```python
from build123d import *

# Parameters (mm, degrees)
SKETCH1_W       = 1193.8
SKETCH1_H       = 1371.6
EXTRUDE1_DEPTH  = 635
EXTRUDE4_DEPTH  = 1270
SKETCH6_W       = 25.4
SKETCH6_H       = 25.4
EXTRUDE5_DEPTH  = 584.2
SKETCH8_W       = 25.4
SKETCH8_H       = 25.4
EXTRUDE6_DEPTH  = 1143
SKETCH9_W       = 25.4
SKETCH9_H       = 25.4
EXTRUDE7_DEPTH  = 584.2
SKETCH10_W      = 25.4
SKETCH10_H      = 25.4
EXTRUDE8_DEPTH  = 1143
SHELL2_T        = -25.4
SKETCH17_R      = 3.175
EXTRUDE14_DEPTH = 1927.050362789
SKETCH24_W      = 1143
SKETCH24_H      = 584.2
EXTRUDE15_DEPTH = 25.4
SKETCH12_W      = 1143
SKETCH12_H      = 76.2
EXTRUDE16_DEPTH = 38.1
SKETCH13_W      = 584.2
SKETCH13_H      = 76.2
EXTRUDE17_DEPTH = 38.1
SKETCH14_W      = 1143
SKETCH14_H      = 76.2
EXTRUDE18_DEPTH = 38.1
SKETCH11_W      = 584.2
SKETCH11_H      = 76.2
EXTRUDE19_DEPTH = 38.1
SKETCH30_W      = 1143
SKETCH30_H      = 5.614753794
EXTRUDE20_DEPTH = 76.2


with BuildPart() as part:
    # Sketch1 → Extrude1 (new body)
    with BuildSketch(Plane.XY):
        with Locations((596.9, 685.8)):
            Rectangle(SKETCH1_W, SKETCH1_H)
    extrude(amount=EXTRUDE1_DEPTH)

    # Sketch2 → Extrude4 (cut)
    with BuildSketch(Plane(origin=(0, 1371.6, 0), x_dir=(1, 0, 0), z_dir=(0, 1, 0))):
        Polygon((25.4, -609.6), (25.4, -635), (1168.4, -635), (1168.4, -609.6), (1193.8, -609.6), (1193.8, -25.4), (1168.4, -25.4), (1168.4, 0), (25.4, 0), (25.4, -25.4), (0, -25.4), (0, -609.6), align=None)
    extrude(amount=-EXTRUDE4_DEPTH, mode=Mode.SUBTRACT)

    # Sketch6 → Extrude5 (add)
    with BuildSketch(Plane.XY.offset(25.4)):
        with Locations((12.7, 1358.9)):
            Rectangle(SKETCH6_W, SKETCH6_H)
    extrude(amount=EXTRUDE5_DEPTH)

    # Sketch8 → Extrude6 (add)
    with BuildSketch(Plane(origin=(25.4, 0, 0), x_dir=(0, 0, -1), z_dir=(1, 0, 0))):
        with Locations((-622.3, 1358.9)):
            Rectangle(SKETCH8_W, SKETCH8_H)
    extrude(amount=EXTRUDE6_DEPTH)

    # Sketch9 → Extrude7 (add)
    with BuildSketch(Plane(origin=(0, 0, 609.6), x_dir=(-1, 0, 0), z_dir=(0, 0, -1))):
        with Locations((-1181.1, 1358.9)):
            Rectangle(SKETCH9_W, SKETCH9_H)
    extrude(amount=EXTRUDE7_DEPTH)

    # Sketch10 → Extrude8 (add)
    with BuildSketch(Plane.ZY.offset(-1168.4)):
        with Locations((12.7, 1358.9)):
            Rectangle(SKETCH10_W, SKETCH10_H)
    extrude(amount=EXTRUDE8_DEPTH)

    # Shell2
    shell2_openings = [part.faces().sort_by_distance(p)[0] for p in [
        (596.9, 0, 317.5),
    ]]
    offset(amount=SHELL2_T, openings=shell2_openings)

    # Sketch17 → Extrude14 (cut, through all)
    with BuildSketch(Plane(origin=(0, 1371.6, 0), x_dir=(1, 0, 0), z_dir=(0, 1, 0))):
        with Locations(Location((1181.1, -622.3, 0), (0, 0, 270))):
            Circle(SKETCH17_R)
        with Locations(Location((1181.1, -12.7, 0), (0, 0, 270))):
            Circle(SKETCH17_R)
        with Locations(Location((12.7, -12.7, 0), (0, 0, 270))):
            Circle(SKETCH17_R)
        with Locations(Location((12.7, -622.3, 0), (0, 0, 270))):
            Circle(SKETCH17_R)
    extrude(amount=-EXTRUDE14_DEPTH, mode=Mode.SUBTRACT)

    # Sketch24 → Extrude15 (cut)
    with BuildSketch(Plane(origin=(0, 101.6, 0), x_dir=(1, 0, 0), z_dir=(0, 1, 0))):
        with Locations((596.9, -317.5)):
            Rectangle(SKETCH24_W, SKETCH24_H)
    extrude(amount=-EXTRUDE15_DEPTH, mode=Mode.SUBTRACT)

    # Sketch12 → Extrude16 (cut)
    with BuildSketch(Plane.XY.offset(25.4)):
        with Locations((596.9, 38.1)):
            Rectangle(SKETCH12_W, SKETCH12_H)
    extrude(amount=-EXTRUDE16_DEPTH, mode=Mode.SUBTRACT)

    # Sketch13 → Extrude17 (cut)
    with BuildSketch(Plane.ZY.offset(-1168.4)):
        with Locations((317.5, 38.1)):
            Rectangle(SKETCH13_W, SKETCH13_H)
    extrude(amount=-EXTRUDE17_DEPTH, mode=Mode.SUBTRACT)

    # Sketch14 → Extrude18 (cut)
    with BuildSketch(Plane(origin=(0, 0, 609.6), x_dir=(-1, 0, 0), z_dir=(0, 0, -1))):
        with Locations((-596.9, 38.1)):
            Rectangle(SKETCH14_W, SKETCH14_H)
    extrude(amount=-EXTRUDE18_DEPTH, mode=Mode.SUBTRACT)

    # Sketch11 → Extrude19 (cut)
    with BuildSketch(Plane(origin=(25.4, 0, 0), x_dir=(0, 0, -1), z_dir=(1, 0, 0))):
        with Locations((-317.5, 38.1)):
            Rectangle(SKETCH11_W, SKETCH11_H)
    extrude(amount=-EXTRUDE19_DEPTH, mode=Mode.SUBTRACT)

    # Sketch30 → Extrude20 (add)
    with BuildSketch(Plane.XZ.offset(-76.2)):
        with Locations((596.9, 622.563749497)):
            Rectangle(SKETCH30_W, SKETCH30_H)
    extrude(amount=EXTRUDE20_DEPTH)


solid = part.part
```
CAD build for the part. Positions are in the model's coordinates, mm. A direction names the side the tool comes from. Coordinates: 2 decimals unless noted, no trailing zeros. Write each loop counter-clockwise with the first axis right and the second up, starting at its lowest first coordinate (ties: lowest second). Pieces come first, ordered by that corner, then holes. Notation, with made-up numbers: (56.25, 74.25) -> (78.25, 74.25) arc R19 cw to (78.25, 99.25) -> close; hole circle Ø4 at (58.25, -3). An arc over 180 degrees is marked (long way). Use CSV: the item, a comma, the result in double quotes. Start each with the question number.
Item 1: Two-plate mould, pull along X, no slides. Class faces 1 (the flat face through (1193.8, 683, 13)), 2 (the flat face through (19, 683, 635)), 3 (the flat face through (589, 39, 625.371)): +X half, -X half, draft (parallel to the pull), parting line (faces both ways), or undercut.
Item 2: Band-saw the part on C-C, the plane z = 175.5. Write the cut outline in (x, y), plus the area to 3 significant figures.
Item 3: Wall check: probe 1 along X at (y, z) = (296.5, 12.7) (3 decimals); probe 2 along Z at (x, y) = (12, 431); probe 3 along Z at (x, y) = (1181.1, 936) (3 decimals). Give the ranges that are in metal, low to high.
Item 4: Drop flat-ended pins along their axis: P1, Ø10.5, axis at y = 21.5, z = 629.5, coming from the -X side; P2, Ø7.5, axis at x = 1182, z = 341, coming from the -Y side. Give the stop position or say it passes through.
Item 5: Band-saw the part on A-A, the plane x = 722.5. Write the cut outline in (y, z), plus the area to 3 significant figures.
Item 6: Band-saw the part on B-B, the plane y = 826.5. Write the cut outline in (x, z) (3 decimals).
Item 7: Tool access for faces 4 (the flat face through (1174, 683, 0)), 5 (the flat face through (589, 39, 619.756)): list every direction of +Z, -Z, +X, -X, +Y, -Y with a clear straight run to the whole face (end or side of a thin tool).
Response values:
1,face 1,"+X half"
1,face 2,"draft"
1,face 3,"undercut"
2,outline,"(0, 76.2) -> (25.4, 76.2) -> (25.4, 101.6) -> (0, 101.6) -> close; (0, 1346.2) -> (25.4, 1346.2) -> (25.4, 1371.6) -> (0, 1371.6) -> close; (1168.4, 76.2) -> (1193.8, 76.2) -> (1193.8, 101.6) -> (1168.4, 101.6) -> close; (1168.4, 1346.2) -> (1193.8, 1346.2) -> (1193.8, 1371.6) -> (1168.4, 1371.6) -> close"
2,area,"2,580 mm2"
3,probe 1,"x = 0 to 9.525, 15.875 to 25.4, 1168.4 to 1177.925, 1184.275 to 1193.8"
3,probe 2,"z = 0 to 9.6, 15.8 to 25.4, 609.6 to 619.2, 625.4 to 635"
3,probe 3,"z = 0 to 9.525, 15.875 to 25.4, 609.6 to 619.125, 625.475 to 635"
4,P1,"stops at x = 0"
4,P2,"stops at y = 76.2"
5,outline,"(0, 619.76) -> (76.2, 619.76) -> (76.2, 609.6) -> (101.6, 609.6) -> (101.6, 635) -> (76.2, 635) -> (76.2, 625.37) -> (0, 625.37) -> close; (76.2, 0) -> (101.6, 0) -> (101.6, 25.4) -> (76.2, 25.4) -> close; (1346.2, 0) -> (1371.6, 0) -> (1371.6, 25.4) -> (1346.2, 25.4) -> close; (1346.2, 609.6) -> (1371.6, 609.6) -> (1371.6, 635) -> (1346.2, 635) -> close"
5,area,"3,010 mm2"
6,outline,"(0, 0) -> (25.4, 0) -> (25.4, 25.4) -> (0, 25.4) -> close; (0, 609.6) -> (25.4, 609.6) -> (25.4, 635) -> (0, 635) -> close; (1168.4, 0) -> (1193.8, 0) -> (1193.8, 25.4) -> (1168.4, 25.4) -> close; (1168.4, 609.6) -> (1193.8, 609.6) -> (1193.8, 635) -> (1168.4, 635) -> close; hole circle Ø6.35 at (12.7, 12.7); hole circle Ø6.35 at (12.7, 622.3); hole circle Ø6.35 at (1181.1, 12.7); hole circle Ø6.35 at (1181.1, 622.3)"
7,face 4,"-Z, +X, -X, +Y, -Y"
7,face 5,"-Z, -Y"
